from build123d import *

# Parameters (mm, degrees)
SKETCH_1_R      = 2.25
EXTRUDE_1_DEPTH = 3


with BuildPart() as part:
    # 草图1 → 凸台-拉伸1 (new body)
    with BuildSketch(Plane(origin=(0, 0, 0), x_dir=(-1, 0, 0), z_dir=(0, 0, -1))):
        with BuildLine():
            Line((-41.791952639, -38.236908366), (-41.547911956, -38.150201988))
            ThreePointArc((-41.547911956, -38.150201988), (-41.297660294, -37.953957018), (-41.216368699, -37.646500259))
            ThreePointArc((-41.216368699, -37.646500259), (-36.850985646, -36.746719128), (-40.805488223, -38.802949817))
            ThreePointArc((-40.805488223, -38.802949817), (-41.062544272, -38.615706205), (-41.380516207, -38.621348105))
            Line((-41.380516207, -38.621348105), (-41.62455689, -38.708054482))
            ThreePointArc((-41.62455689, -38.708054482), (-41.932143393, -39.023021663), (-41.871497469, -39.459067365))
            ThreePointArc((-41.871497469, -39.459067365), (-41.243343249, -40.162162054), (-40.450307086, -40.672077255))
            Line((-40.450307086, -40.672077255), (-37.864755045, -41.877739972))
            ThreePointArc((-37.864755045, -41.877739972), (-37.116075694, -41.916780886), (-36.550657336, -41.424493323))
            ThreePointArc((-36.550657336, -41.424493323), (0, -19), (36.550657336, -41.424493323))
            ThreePointArc((36.550657336, -41.424493323), (37.116075694, -41.916780886), (37.864755045, -41.877739972))
            Line((37.864755045, -41.877739972), (40.450307086, -40.672077255))
            ThreePointArc((40.450307086, -40.672077255), (41.243343249, -40.162162054), (41.871497469, -39.459067365))
            ThreePointArc((41.871497469, -39.459067365), (41.932143393, -39.023021663), (41.62455689, -38.708054482))
            Line((41.62455689, -38.708054482), (41.380516207, -38.621348105))
            ThreePointArc((41.380516207, -38.621348105), (41.062544272, -38.615706205), (40.805488223, -38.802949817))
            ThreePointArc((40.805488223, -38.802949817), (36.850985646, -36.746719128), (41.216368699, -37.646500259))
            ThreePointArc((41.216368699, -37.646500259), (41.297660294, -37.953957018), (41.547911956, -38.150201988))
            Line((41.547911956, -38.150201988), (41.791952639, -38.236908366))
            ThreePointArc((41.791952639, -38.236908366), (42.229313556, -38.186617104), (42.457382592, -37.810055957))
            ThreePointArc((42.457382592, -37.810055957), (42.413654712, -36.868245075), (42.120121371, -35.972277417))
            ThreePointArc((42.120121371, -35.972277417), (38.193299638, -29.507864773), (33.125428162, -23.893130722))
            ThreePointArc((33.125428162, -23.893130722), (26.210916767, -14.399107105), (23.515754966, -2.967438148))
            ThreePointArc((23.515754966, -2.967438148), (23.211784398, -2.281473086), (22.516285244, -2))
            Line((22.516285244, -2), (-22.516285244, -2))
            ThreePointArc((-22.516285244, -2), (-23.211784398, -2.281473086), (-23.515754966, -2.967438148))
            ThreePointArc((-23.515754966, -2.967438148), (-26.210916767, -14.399107105), (-33.125428162, -23.893130722))
            ThreePointArc((-33.125428162, -23.893130722), (-38.193299638, -29.507864773), (-42.120121371, -35.972277417))
            ThreePointArc((-42.120121371, -35.972277417), (-42.413654712, -36.868245075), (-42.457382592, -37.810055957))
            ThreePointArc((-42.457382592, -37.810055957), (-42.229313556, -38.186617104), (-41.791952639, -38.236908366))
        make_face()
        with Locations(Location((0, -6, 0), (0, 0, 180))):
            Circle(SKETCH_1_R, mode=Mode.SUBTRACT)
        with Locations(Location((19.5, -6, 0), (0, 0, 180))):
            Circle(SKETCH_1_R, mode=Mode.SUBTRACT)
        with Locations(Location((-19.5, -6, 0), (0, 0, 180))):
            Circle(SKETCH_1_R, mode=Mode.SUBTRACT)
    extrude(amount=-EXTRUDE_1_DEPTH)


solid = part.part
Source: CAD feature listing. Evaluate the final solid. Frame: model axes, mm. Round coordinates to 2 decimals unless told otherwise and drop trailing zeros. Loops run counter-clockwise (first coordinate to the right, second up) from the corner with the lowest first, then second, coordinate; pieces in that order, holes last. Notation, with made-up numbers: (79, 16) -> (124, 16) arc R15 ccw to (124, 24) -> close; hole circle Ø5 at (55.5, 51.25). An arc over 180 degrees is marked (long way). Answer as a JSON object with one key per item and string values. Group by question number.
Q1. Ray query, line 1 (X direction, y = -5.5, z = 2.55); line 2 (X direction, y = -37.5, z = 2.5); line 3 (Y direction, x = 19.5, z = 1.25). Return the intervals inside material, ascending. Write a range as from..to.
Q2. Mould query, pull axis Y, two halves, no side actions, for faces 1 (the cylindrical face through (42.411, -36.855, 1.479)), 2 (the cylindrical face through (38.13, -29.42, 1.48)), 3 (the cylindrical face through (41.253, -40.154, 1.479)), 4 (the cylindrical face through (-36.822, -36.832, 1.479)). Classes: pulls with the +Y half, pulls with the -Y half, needs draft (parallel to the pull), parting line crosses it, or undercut.
Q3. Section query C-C (z = 2.05). State how many separate pieces and enclosed holes the cut face has, plus the area to 3 significant figures.
Q4. Section query D-D (y = -6). Output: boundary loops of the cut face in (x, z).
Q5. Section query A-A (x = 0). Output: boundary loops of the cut face in (y, z), plus the area to 3 significant figures.
Q6. Section query B-B (y = -34). Output: boundary loops of the cut face in (x, z) (3 decimals), plus the area to 3 significant figures.
Completed:
{
 "1": {"line 1": "-23.71..-21.69, -17.31..-2.19, 2.19..17.31, 21.69..23.71", "line 2": "-42.47..-41.22, -36.72..-34.27, 34.27..36.72, 41.22..42.47", "line 3": "-23.93..-8.25, -3.75..-2"},
 "2": {"face 1": "parting line crosses it", "face 2": "pulls with the +Y half", "face 3": "pulls with the -Y half", "face 4": "undercut"},
 "3": {"separate pieces": "1", "enclosed holes": "3", "area": "1,290 mm²"},
 "4": {"outline": "(-23.77, 0) -> (-21.75, 0) -> (-21.75, 3) -> (-23.77, 3) -> close; (-17.25, 0) -> (-2.25, 0) -> (-2.25, 3) -> (-17.25, 3) -> close; (2.25, 0) -> (17.25, 0) -> (17.25, 3) -> (2.25, 3) -> close; (21.75, 0) -> (23.77, 0) -> (23.77, 3) -> (21.75, 3) -> close"},
 "5": {"outline": "(-19, 0) -> (-8.25, 0) -> (-8.25, 3) -> (-19, 3) -> close; (-3.75, 0) -> (-2, 0) -> (-2, 3) -> (-3.75, 3) -> close", "area": "37.5 mm²"},
 "6": {"outline": "(-41.095, 0) -> (-31.702, 0) -> (-31.702, 3) -> (-41.095, 3) -> close; (31.702, 0) -> (41.095, 0) -> (41.095, 3) -> (31.702, 3) -> close", "area": "56.4 mm²"}
}
